```python
from build123d import *

# Parameters (mm, degrees)
SKETCH4_W           = 13.5
SKETCH4_H           = 13.5
SKETCH4_R           = 2.5
HOLE_TOPMAIN_DEPTH  = 64.27
SKETCH14_R          = 2.5
CUT_EXTRUDE9_DEPTH  = 67.220336
SKETCH15_R          = 3.25
CUT_EXTRUDE10_DEPTH = 66.384500568
SKETCH18_W          = 13.5
SKETCH18_H          = 64.27
SKETCH18_R          = 3.25
BOSS_EXTRUDE2_DEPTH = 13.5
FILLET3_R           = 2
SKETCH19_R          = 2.5
CUT_EXTRUDE11_DEPTH = 13.5
SKETCH22_W          = 13.5
SKETCH22_H          = 64.27
BOSS_EXTRUDE3_DEPTH = 13.5
BOSS_EXTRUDE5_START = -27
SKETCH24_R          = 3.25
BOSS_EXTRUDE5_DEPTH = 27
CUT_EXTRUDE12_START = -64.27
SKETCH25_R          = 2.5
CUT_EXTRUDE12_DEPTH = 64.27
SKETCH26_R          = 2.5
CUT_EXTRUDE13_DEPTH = 13.5
SKETCH28_R          = 2.5
CUT_EXTRUDE14_DEPTH = 13.5
FILLET4_R           = 2
SKETCH29_R          = 2.5
BOSS_EXTRUDE6_DEPTH = 20


with BuildPart() as part:
    # Sketch4 → hole-TopMain (new body)
    with BuildSketch(Plane(origin=(0, 0, 0), x_dir=(1, 0, 0), z_dir=(0, 1, 0))):
        with Locations((-1.75, 1.75)):
            Rectangle(SKETCH4_W, SKETCH4_H)
        with Locations(Location((0, 0, 0), (0, 0, 90))):
            Circle(SKETCH4_R, mode=Mode.SUBTRACT)
    extrude(amount=HOLE_TOPMAIN_DEPTH)

    # Sketch14 → Cut-Extrude9 (cut, through all)
    with BuildSketch(Plane(origin=(0, 0, -8.5), x_dir=(-1, 0, 0), z_dir=(0, 0, -1))):
        with Locations((1.75, 46.135)):
            Circle(SKETCH14_R)
    extrude(amount=-CUT_EXTRUDE9_DEPTH, mode=Mode.SUBTRACT)

    # Sketch15 → Cut-Extrude10 (cut, through all)
    with BuildSketch(Plane(origin=(0, 0, -3.5), x_dir=(-1, 0, 0), z_dir=(0, 0, -1))):
        with Locations((1.75, 46.135)):
            Circle(SKETCH15_R)
    extrude(amount=-CUT_EXTRUDE10_DEPTH, mode=Mode.SUBTRACT)

    # Sketch18 → Boss-Extrude2 (add)
    with BuildSketch(Plane.XY.offset(5)):
        with Locations((-1.75, 32.135)):
            Rectangle(SKETCH18_W, SKETCH18_H)
        with Locations(Location((-1.75, 46.135, 0), (0, 0, 180))):
            Circle(SKETCH18_R, mode=Mode.SUBTRACT)
    extrude(amount=BOSS_EXTRUDE2_DEPTH)

    # Fillet3
    fillet3_edges = [part.edges().sort_by_distance(p)[0] for p in [
        (-8.5, 32.135, -8.5),
        (5, 32.135, 18.5),
    ]]
    fillet(fillet3_edges, radius=FILLET3_R)

    # Sketch19 → Cut-Extrude11 (cut)
    with BuildSketch(Plane.ZY.offset(8.5)):
        with Locations((11.75, 46.135)):
            Circle(SKETCH19_R)
    extrude(amount=-CUT_EXTRUDE11_DEPTH, mode=Mode.SUBTRACT)

    # Sketch22 → Boss-Extrude3 (add)
    with BuildSketch(Plane(origin=(5, 0, 0), x_dir=(0, 0, -1), z_dir=(1, 0, 0))):
        with Locations((1.75, 32.135)):
            Rectangle(SKETCH22_W, SKETCH22_H)
    extrude(amount=BOSS_EXTRUDE3_DEPTH)

    # Sketch24 → Boss-Extrude5 (add)
    with BuildSketch(Plane.XY.offset(18.5).offset(BOSS_EXTRUDE5_START)):
        with Locations((-1.75, 46.135)):
            Circle(SKETCH24_R)
    extrude(amount=BOSS_EXTRUDE5_DEPTH)

    # Sketch25 → Cut-Extrude12 (cut)
    with BuildSketch(Plane(origin=(0, 64.27, 0), x_dir=(1, 0, 0), z_dir=(0, 1, 0)).offset(CUT_EXTRUDE12_START)):
        with Locations(Location((0, 0, 0), (0, 0, 90))):
            Circle(SKETCH25_R)
    extrude(amount=CUT_EXTRUDE12_DEPTH, mode=Mode.SUBTRACT)

    # Sketch26 → Cut-Extrude13 (cut)
    with BuildSketch(Plane.ZY.offset(8.5)):
        with Locations((11.75, 46.135)):
            Circle(SKETCH26_R)
    extrude(amount=-CUT_EXTRUDE13_DEPTH, mode=Mode.SUBTRACT)

    # Sketch28 → Cut-Extrude14 (cut)
    with BuildSketch(Plane(origin=(0, 0, -8.5), x_dir=(-1, 0, 0), z_dir=(0, 0, -1))):
        with Locations((-11.75, 46.135)):
            Circle(SKETCH28_R)
    extrude(amount=-CUT_EXTRUDE14_DEPTH, mode=Mode.SUBTRACT)

    # Fillet4
    fillet4_edges = [part.edges().sort_by_distance(p)[0] for p in [
        (18.5, 32.135, 5),
    ]]
    fillet(fillet4_edges, radius=FILLET4_R)

    # Sketch29 → Boss-Extrude6 (add)
    with BuildSketch(Plane(origin=(0, 64.27, 0), x_dir=(1, 0, 0), z_dir=(0, 1, 0))):
        with BuildLine():
            Line((5, -16.5), (5, -5))
            Line((5, -5), (16.5, -5))
            ThreePointArc((16.5, -5), (17.914213562, -4.414213562), (18.5, -3))
            Line((18.5, -3), (18.5, 8.5))
            Line((18.5, 8.5), (-6.5, 8.5))
            ThreePointArc((-6.5, 8.5), (-7.914213562, 7.914213562), (-8.5, 6.5))
            Line((-8.5, 6.5), (-8.5, -18.5))
            Line((-8.5, -18.5), (3, -18.5))
            ThreePointArc((3, -18.5), (4.414213562, -17.914213562), (5, -16.5))
        make_face()
        with Locations(Location((0, 0, 0), (0, 0, 90))):
            Circle(SKETCH29_R, mode=Mode.SUBTRACT)
    extrude(amount=BOSS_EXTRUDE6_DEPTH)


solid = part.part
```
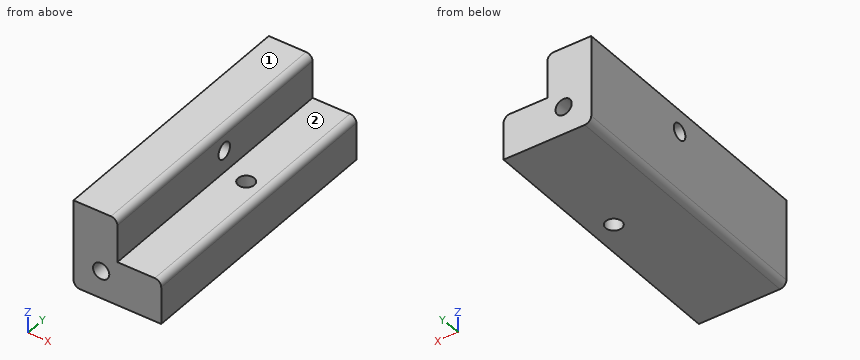
Read the model definition and answer for the solid it produces. Units are mm, in the model's axes. Face numbers are marked on the shaded views. A direction names the side the tool comes from. Round coordinates to 2 decimals unless told otherwise and drop trailing zeros. Write each loop counter-clockwise with the first axis right and the second up, starting at its lowest first coordinate (ties: lowest second). Pieces come first, ordered by that corner, then holes. Notation, with made-up numbers: (-1.5, -32) -> (22.5, -32) arc R27 ccw to (22.5, -2) -> close; hole circle Ø8 at (84, -5.75). An arc over 180 degrees is marked (long way). Answer in a Markdown table with one row per item. Add a question column.
1) Find section A-A, the plane z = 0. Determine the outline of the cut face in (x, y) (3 decimals).
2) Find section B-B, the plane x = 11.75. Determine the outline of the cut face in (y, z) (3 decimals).
3) Consider line 1 (Y direction, x = 11.75, z = -0.25) (3 decimals); line 2 (X direction, y = 21.5, z = 0); line 3 (Z direction, x = 0.25, y = 78). Determine where each line is inside the solid, lowest interval first.
4) Find section D-D, the plane z = 13. Determine the outline of the cut face in (x, y).
5) Given P1, Ø3, axis at x = 8.5, y = 18.5, coming from the +Z side; P2, Ø4, axis at x = 0, z = 0, coming from the -Y side; P3, Ø3.5, axis at y = 56, z = 9.5, coming from the +X side; P4, Ø3, axis at x = 5.5, y = 55.5, coming from the +Z side, each flat-ended and moving along its own axis, determine where each tip first touches the part or whether it passes through.
6) Find section C-C, the plane y = 75. Determine the outline of the cut face in (x, z), and give its area (3 significant figures).
7) Which of the six approach directions +Z, -Z, +X, -X, +Y, -Y give full straight-line access (tool end or side, diameter ignored) to the marked faces 1 and 2?
Findings below:
| question | item | result |
|---|---|---|
| 1 | outline | (-8.5, 0) -> (-2.5, 0) -> (-2.5, 84.27) -> (-8.5, 84.27) -> close; (2.5, 0) -> (18.5, 0) -> (18.5, 84.27) -> (2.5, 84.27) -> close; hole circle Ø5 at (11.75, 46.135) |
| 2 | outline | (0, -8.5) -> (43.635, -8.5) -> (43.635, 5) -> (0, 5) -> close; (48.635, -8.5) -> (84.27, -8.5) -> (84.27, 5) -> (48.635, 5) -> close |
| 3 | line 1 | 0 to 43.635, 48.635 to 84.27 |
| 3 | line 2 | -8.5 to -2.5, 2.5 to 18.5 |
| 3 | line 3 | -8.5 to -2.49, 2.49 to 18.5 |
| 4 | outline | (-8.5, 0) -> (5, 0) -> (5, 43.97) -> (-8.5, 43.97) -> close; (-8.5, 48.3) -> (5, 48.3) -> (5, 84.27) -> (-8.5, 84.27) -> close |
| 5 | P1 | z = 5 |
| 5 | P2 | through |
| 5 | P3 | x = 5 |
| 5 | P4 | z = 18.23 |
| 6 | outline | (-8.5, -6.5) arc R2 ccw to (-6.5, -8.5) -> (18.5, -8.5) -> (18.5, 3) arc R2 ccw to (16.5, 5) -> (5, 5) -> (5, 16.5) arc R2 ccw to (3, 18.5) -> (-8.5, 18.5) -> close; hole circle Ø5 at (0, 0) |
| 6 | area | 525 mm² |
| 7 | face 1 | +Z, +X, -X, +Y, -Y |
| 7 | face 2 | +Z, +X, +Y, -Y |
